Geometry: see drawing. Coordinates: mm, zero at the bounding-box minimum. A direction names the side the tool comes from. Round coordinates to 2 decimals unless told otherwise and drop trailing zeros. Order: outer loops, then holes, each group sorted by start corner. A loop starts at its lowest first (then second) coordinate and runs counter-clockwise, first axis right, second up. Notation, with made-up numbers: (12.25, 0.25) -> (69.25, 0.25) arc R9 cw to (69.25, 8.25) -> close; hole circle Ø10 at (66, -8). An arc over 180 degrees is marked (long way). Answer as CSV lines item,"result". Start each with the question number.
(1) Line query: line 1 along Y through (x, z) = (1.5, 12); line 2 along Y through (x, z) = (8, 40.7); line 3 along Z through (x, y) = (6.5, 9). Output: solid intervals per line, ascending. Write a range as from..to.
(2) Set-up query: the marked faces 1 and 2. Return all of +Z, -Z, +X, -X, +Y, -Y with unobstructed straight access to the full face (end or side cutting, diameter ignored); none if empty.
(3) Section query A-A (x = 8). Output: boundary loops of the cut face in (y, z), plus the area to 3 significant figures.
(4) Section query C-C (y = 40). Output: boundary loops of the cut face in (x, z).
(5) Contact query for flat-ended pins moving along their axis: P1, Ø4, axis at y = 31.5, z = 33, coming from the +X side; P2, Ø4, axis at x = 1.5, y = 8.5, coming from the -Z side; P3, Ø2.5, axis at x = 6.5, y = 30.5, coming from the -Z side. Output: stop coordinate, or through.
(6) Section query B-B (y = 33). Output: boundary loops of the cut face in (x, z), plus the area to 3 significant figures.
(7) Section query D-D (z = 24). Output: boundary loops of the cut face in (x, y).
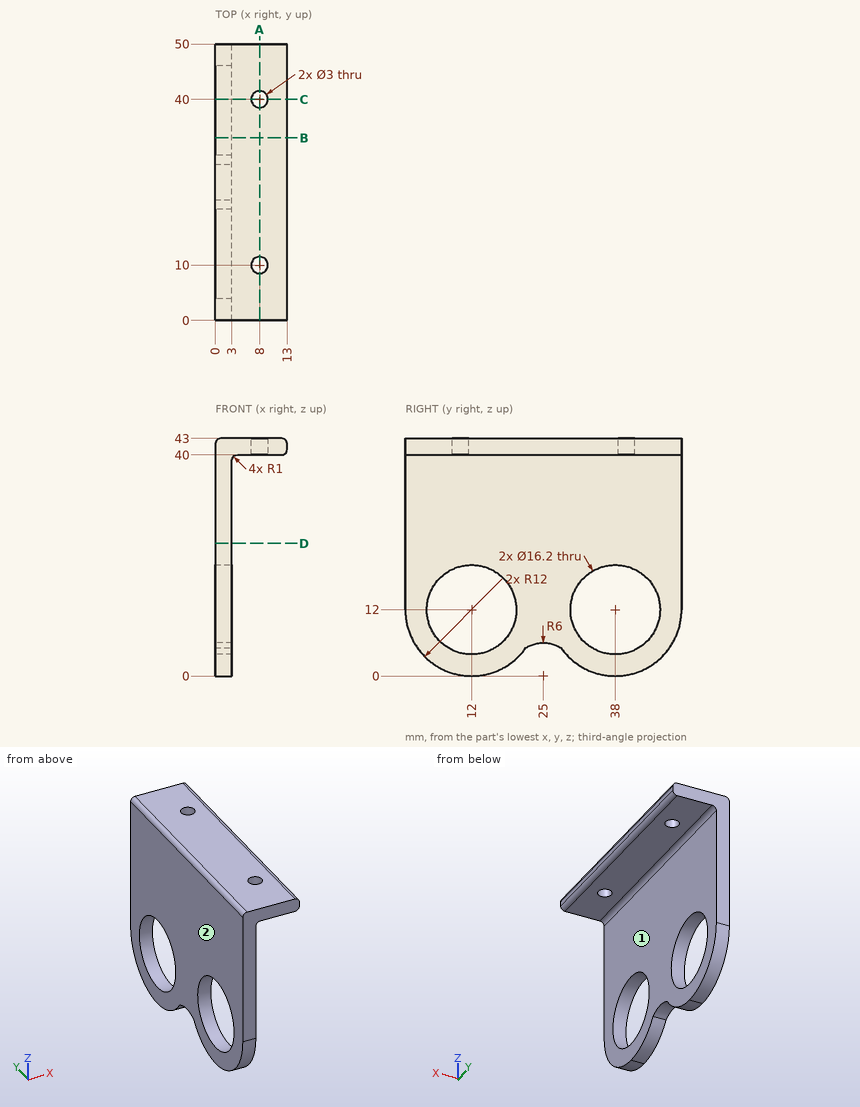
Answer block:
1,line 1,"0..3.9, 20.1..29.9, 46.1..50"
1,line 2,"0..8.5, 11.5..38.5, 41.5..50"
1,line 3,"40..43"
2,face 1,"-Z, +X, +Y, -Y"
2,face 2,"+Z, -Z, -X, +Y, -Y"
3,outline,"(0, 40) -> (8.5, 40) -> (8.5, 43) -> (0, 43) -> close; (11.5, 40) -> (38.5, 40) -> (38.5, 43) -> (11.5, 43) -> close; (41.5, 40) -> (50, 40) -> (50, 43) -> (41.5, 43) -> close"
3,area,"132 mm2"
4,outline,"(0, 0.17) -> (3, 0.17) -> (3, 4.15) -> (0, 4.15) -> close; (0, 19.85) -> (3, 19.85) -> (3, 39) arc R1 cw to (4, 40) -> (6.5, 40) -> (6.5, 43) -> (1, 43) arc R1 ccw to (0, 42) -> close; (9.5, 40) -> (12, 40) arc R1 ccw to (13, 41) -> (13, 42) arc R1 ccw to (12, 43) -> (9.5, 43) -> close"
5,P1,"x = 3"
5,P2,"z = 0.09"
5,P3,"z = 40"
6,outline,"(0, 1.09) -> (3, 1.09) -> (3, 5.63) -> (0, 5.63) -> close; (0, 18.37) -> (3, 18.37) -> (3, 39) arc R1 cw to (4, 40) -> (12, 40) arc R1 ccw to (13, 41) -> (13, 42) arc R1 ccw to (12, 43) -> (1, 43) arc R1 ccw to (0, 42) -> close"
6,area,"117 mm2"
7,outline,"(0, 0) -> (3, 0) -> (3, 50) -> (0, 50) -> close"
